Study the drawing (mm; zero at the part's minimum x, y, z) and answer. A direction names the side the tool comes from. Coordinates: 2 decimals unless noted, no trailing zeros. Loops run counter-clockwise (first coordinate to the right, second up) from the corner with the lowest first, then second, coordinate; pieces in that order, holes last.
Q1. Straight lines are drawn through the part: line 1 (Y direction, x = 60, z = 51); line 2 (X direction, y = 32, z = 51) (1 decimal); line 3 (X direction, y = 46, z = 20) (1 decimal). For each, find the intervals that lie inside material, in ascending order.
Q2. Section C-C (z = 24.5) is taken. Give the vertices of the cut face in (x, y).
Q3. Flat-ended cylindrical pins translate along their axes: P1, Ø2, axis at y = 38, z = 22, coming from the -X side (1 decimal); P2, Ø6, axis at y = 82.5, z = 33, coming from the -X side; P3, Ø1, axis at x = 96, z = 39, coming from the -Y side. Find the tip coordinate at first contact, or state that the pin passes through.
Q4. Section B-B (y = 60) is taken. Give the vertices of the cut face in (x, z), then the cut area to 4 significant figures.
Q5. The mould has two halves that part along Y. Classify the marked faces 1, 2 and 3: pulls with the +Y half, pulls with the -Y half, needs draft (parallel to the pull), parting line crosses it, or undercut.
Q6. Which of the six approach directions +Z, -Z, +X, -X, +Y, -Y give full straight-line access (tool end or side, diameter ignored) to the marked faces 4, 5 and 6?
Q7. Section A-A (x = 60) is taken. Give the vertices of the cut face in (y, z), then the cut area to 3 significant figures.
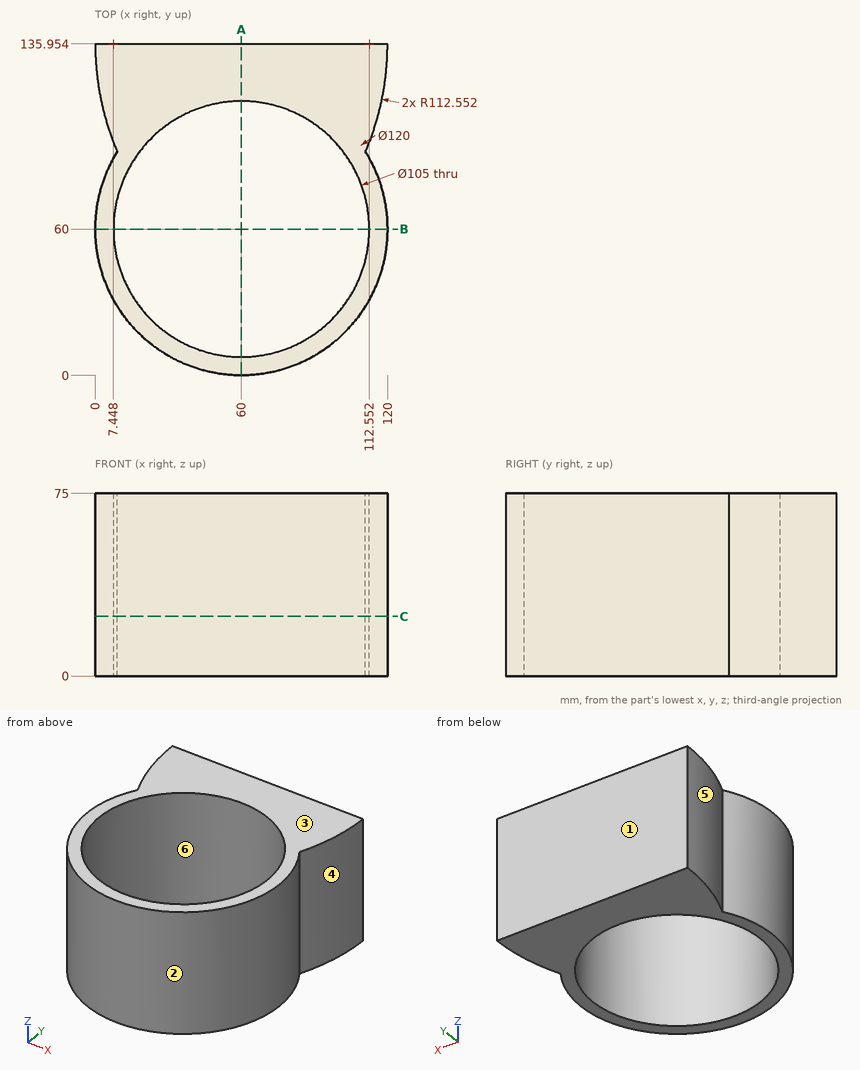
Numbers:
1. line 1: y = 0 to 7.5, 112.5 to 135.95
1. line 2: x = 6.9 to 15.6, 104.4 to 113.1
1. line 3: x = 1.7 to 9.4, 110.6 to 118.3
2. outline: (0, 135.95) arc R112.55 ccw to (9.06, 91.71) arc R60 ccw (long way) to (110.94, 91.71) arc R112.55 ccw to (120, 135.95) - close; hole circle Ø105 at (60, 60)
3. P1: stops at x = 3.8
3. P2: stops at x = 3.26
3. P3: stops at y = 11.63
4. outline: (0, 0) - (7.5, 0) - (7.5, 75) - (0, 75) - close; (112.5, 0) - (120, 0) - (120, 75) - (112.5, 75) - close
4. area: 1,125 mm2
5. face 1: pulls with the +Y half
5. face 2: undercut
5. face 3: needs draft
6. face 4: +Z, -Z, +X
6. face 5: +Z, -Z, -X
6. face 6: +Z, -Z
7. outline: (0, 0) - (7.5, 0) - (7.5, 75) - (0, 75) - close; (112.5, 0) - (135.95, 0) - (135.95, 75) - (112.5, 75) - close
7. area: 2,320 mm2
